For this review, take the finished solid that the model builds, in its own axes (mm). Face numbers are marked on the shaded views. A direction names the side the tool comes from. Give positions to 0.01 mm unless a question says otherwise; leave off trailing zeros. Loops run counter-clockwise (first coordinate to the right, second up) from the corner with the lowest first, then second, coordinate; pieces in that order, holes last. Notation, with made-up numbers: (7, -29) - (20, -29) arc R24 cw to (20, -13) - close; hole circle Ø2 at (28, 79). An arc over 180 degrees is marked (long way). Put each result on its own line as item: value. Start each with the question number.
from build123d import *

# Parameters (mm, degrees)
SKETCH2_W           = 69.99986
SKETCH2_H           = 31.999936
BOSS_EXTRUDE1_DEPTH = 1.6
SKETCH3_R           = 5.533230125
SKETCH3_W           = 8.0009746
SKETCH3_H           = 15.8759652
SKETCH3_W_2         = 9.1719654
SKETCH3_H_2         = 3.5780218
BOSS_EXTRUDE2_DEPTH = 7.5
SKETCH4_R           = 4.745015856
BOSS_EXTRUDE3_DEPTH = 12


with BuildPart() as part:
    # Sketch2 → Boss-Extrude1 (new body)
    with BuildSketch(Plane.XY):
        with Locations((34.99993, 15.999968)):
            Rectangle(SKETCH2_W, SKETCH2_H)
    extrude(amount=-BOSS_EXTRUDE1_DEPTH)

    # Sketch3 → Boss-Extrude2 (add)
    with BuildSketch(Plane.XY):
        with Locations((51.999892991, 23.999962155)):
            Circle(SKETCH3_R)
        with Locations((65.5473543, 17.999964)):
            Rectangle(SKETCH3_W, SKETCH3_H)
        with Locations((4.4525057, 17.999964)):
            Rectangle(SKETCH3_W, SKETCH3_H)
        with Locations((36.9859433, 24.0110899)):
            Rectangle(SKETCH3_W_2, SKETCH3_H_2)
    extrude(amount=BOSS_EXTRUDE2_DEPTH)

    # Sketch4 → Boss-Extrude3 (add)
    with BuildSketch(Plane.XY.offset(7.5)):
        with Locations((51.999892991, 23.999962155)):
            Circle(SKETCH4_R)
    extrude(amount=BOSS_EXTRUDE3_DEPTH)


solid = part.part
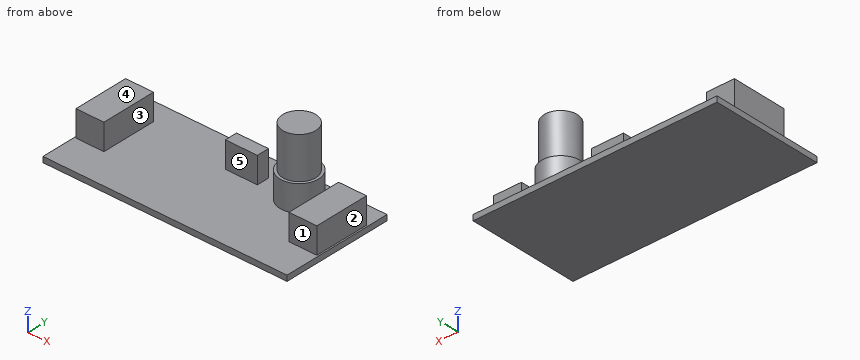
1) Take a section at D-D on x = 38. State the section outline as (y, z) points, and give its area (3 significant figures).
2) Take a section at C-C on z = 5.75. State the section outline as (x, y) points, and give its area (3 significant figures).
3) Take a section at B-B on y = 13.5. State the section outline as (x, z) points.
4) Wall thickness on probe 1 along X at (y, z) = (24.5, 1.5); probe 2 along X at (y, z) = (21.5, 0.25); probe 3 along Z at (x, y) = (6, 30): over which ranges is each line inside the solid? List them lowest first.
5) Take a section at A-A on x = 6. State the section outline as (y, z) points.
6) Machinability: for the marked faces 1, 2, 3, 4 and 5, which of the approach directions +Z, -Z, +X, -X, +Y, -Y give a long, thin tool a straight path to every point of the face, cutting with its end or side? Answer none if there is none.
7) Insertion check: P1, Ø4, axis at x = 66.5, z = 3.5, coming from the -Y side; P2, Ø1.1, axis at x = 36, y = 23.5, coming from the +Z side; P3, Ø6, axis at y = 17, z = 5, coming from the +X side. Each pin has a flat end and moves straight along its axis. Give the tip position at first contact, or say it passes through.
Answers follow:
1. outline: (0, -1.6) - (32, -1.6) - (32, 0) - (25.8, 0) - (25.8, 7.5) - (22.22, 7.5) - (22.22, 0) - (0, 0) - close
1. area: 78.0 mm2
2. outline: (0.45, 10.06) - (8.45, 10.06) - (8.45, 25.94) - (0.45, 25.94) - close; (32.4, 22.22) - (41.57, 22.22) - (41.57, 25.8) - (32.4, 25.8) - close; circle Ø11.07 at (52, 24); (61.55, 10.06) - (69.55, 10.06) - (69.55, 25.94) - (61.55, 25.94) - close
2. area: 383 mm2
3. outline: (0, -1.6) - (70, -1.6) - (70, 0) - (69.55, 0) - (69.55, 7.5) - (61.55, 7.5) - (61.55, 0) - (8.45, 0) - (8.45, 7.5) - (0.45, 7.5) - (0.45, 0) - (0, 0) - close
4. probe 1: 0.45 to 8.45, 32.4 to 41.57, 46.49 to 57.51, 61.55 to 69.55
4. probe 2: 0.45 to 8.45, 47.06 to 56.94, 61.55 to 69.55
4. probe 3: -1.6 to 0
5. outline: (0, -1.6) - (32, -1.6) - (32, 0) - (25.94, 0) - (25.94, 7.5) - (10.06, 7.5) - (10.06, 0) - (0, 0) - close
6. face 1: +Z, +X, -X, -Y
6. face 2: +Z, +X, +Y, -Y
6. face 3: +Z, +Y, -Y
6. face 4: +Z, -X, +Y, -Y
6. face 5: +Z, -Y
7. P1: y = 10.06
7. P2: z = 7.5
7. P3: x = 69.55
